Read the model definition and answer for the solid it produces. Units are mm, in the model's axes. Face numbers are marked on the shaded views. A direction names the side the tool comes from. Round coordinates to 2 decimals unless told otherwise and drop trailing zeros. Loops run counter-clockwise (first coordinate to the right, second up) from the corner with the lowest first, then second, coordinate; pieces in that order, holes last. Notation, with made-up numbers: (-14, -30.75) -> (8, -30.75) arc R25 ccw to (8, -17.75) -> close; hole circle Ø4 at (-25.5, 13.25). An arc over 180 degrees is marked (long way). Put each result on its own line as item: value.
from build123d import *

# Parameters (mm, degrees)
ESQUISSE1_W             = 77
ESQUISSE1_H             = 60
BOSS_EXTRU_1_DEPTH      = 3
BOSS_EXTRU_2_DEPTH      = 50
ESQUISSE3_W             = 55.4
ESQUISSE3_H             = 3
BOSS_EXTRU_3_DEPTH      = 74
ENL_V_MAT_EXTRU_2_REACH = 113.077
ESQUISSE5_R             = 5
BOSS_EXTRU_5_DEPTH      = 48
ENL_V_MAT_EXTRU_3_REACH = 113.077
ESQUISSE8_W             = 5
ESQUISSE8_H             = 10
ENL_V_MAT_EXTRU_4_DEPTH = 5
ESQUISSE10_R            = 5
ENL_V_MAT_EXTRU_5_DEPTH = 3
ESQUISSE11_W            = 74
ESQUISSE11_H            = 60
ENL_V_MAT_EXTRU_6_DEPTH = 5


with BuildPart() as part:
    # Esquisse1 → Boss.-Extru.1 (new body)
    with BuildSketch(Plane(origin=(0, 0, 0), x_dir=(1, 0, 0), z_dir=(0, 1, 0))):
        with Locations((38.5, 30)):
            Rectangle(ESQUISSE1_W, ESQUISSE1_H)
    extrude(amount=BOSS_EXTRU_1_DEPTH)

    # Esquisse2 → Boss.-Extru.2 (add)
    with BuildSketch(Plane(origin=(0, 3, 0), x_dir=(1, 0, 0), z_dir=(0, 1, 0))):
        Polygon((0, 60), (77, 60), (77, 0), (0, 0), (0, 2.3), (74, 2.3), (74, 57.7), (0, 57.7), align=None)
    extrude(amount=BOSS_EXTRU_2_DEPTH)

    # Esquisse3 → Boss.-Extru.3 (add)
    with BuildSketch(Plane.ZY.offset(-74)):
        with Locations((-30, 51.5)):
            Rectangle(ESQUISSE3_W, ESQUISSE3_H)
    extrude(amount=BOSS_EXTRU_3_DEPTH)

    # Esquisse5 → Enlèv. mat.-Extru.2 (cut, up to next)
    with BuildSketch(Plane(origin=(0, 0, -60), x_dir=(-1, 0, 0), z_dir=(0, 0, -1)), mode=Mode.PRIVATE) as enl_v_mat_extru_2_sk1:
        with Locations((-39, 29)):
            Circle(ESQUISSE5_R)
    enl_v_mat_extru_2_tool1 = extrude(enl_v_mat_extru_2_sk1.sketch, amount=-ENL_V_MAT_EXTRU_2_REACH, mode=Mode.PRIVATE) & part.part
    # Esquisse5 → Enlèv. mat.-Extru.2 (cut, up to next)
    with BuildSketch(Plane(origin=(0, 0, -60), x_dir=(-1, 0, 0), z_dir=(0, 0, -1)), mode=Mode.PRIVATE) as enl_v_mat_extru_2_sk2:
        with Locations((-10, 40.5)):
            Circle(ESQUISSE5_R)
    enl_v_mat_extru_2_tool2 = extrude(enl_v_mat_extru_2_sk2.sketch, amount=-ENL_V_MAT_EXTRU_2_REACH, mode=Mode.PRIVATE) & part.part
    add(enl_v_mat_extru_2_tool1.solids().sort_by_distance((39, 29, -60))[0], mode=Mode.SUBTRACT)
    add(enl_v_mat_extru_2_tool2.solids().sort_by_distance((10, 40.5, -60))[0], mode=Mode.SUBTRACT)

    # Esquisse7 → Boss.-Extru.5 (add)
    with BuildSketch(Plane.XZ):
        Polygon((0, 0), (-4.8, 0), (-4.8, -4.8), (-2.5, -4.8), (-2.5, -2.3), (0, -2.3), align=None)
        Polygon((0, -57.7), (0, -60), (-4.8, -60), (-4.8, -55.2), (-2.5, -55.2), (-2.5, -57.7), align=None)
    extrude(amount=-BOSS_EXTRU_5_DEPTH)

    # Esquisse8 → Enlèv. mat.-Extru.3 (cut, up to next)
    with BuildSketch(Plane(origin=(0, 53, 0), x_dir=(1, 0, 0), z_dir=(0, 1, 0)), mode=Mode.PRIVATE) as enl_v_mat_extru_3_sk1:
        with Locations((2.5, 30)):
            Rectangle(ESQUISSE8_W, ESQUISSE8_H)
    enl_v_mat_extru_3_tool1 = extrude(enl_v_mat_extru_3_sk1.sketch, amount=-ENL_V_MAT_EXTRU_3_REACH, mode=Mode.PRIVATE) & part.part
    add(enl_v_mat_extru_3_tool1.solids().sort_by_distance((2.5, 53, -30))[0], mode=Mode.SUBTRACT)

    # Esquisse9 → Enlèv. mat.-Extru.4 (cut)
    with BuildSketch(Plane.XZ):
        Polygon((0, -2.3), (-2.5, -2.3), (-2.5, -4.8), (-4.8, -4.8), (-4.8, 0), (0, 0), align=None)
        Polygon((0, -60), (0, -57.7), (-2.5, -57.7), (-2.5, -55.2), (-4.8, -55.2), (-4.8, -60), align=None)
    extrude(amount=-ENL_V_MAT_EXTRU_4_DEPTH, mode=Mode.SUBTRACT)

    # Esquisse10 → Enlèv. mat.-Extru.5 (cut)
    with BuildSketch(Plane.XY):
        with Locations((10, 12.5)):
            Circle(ESQUISSE10_R)
        with Locations((39, 24)):
            Circle(ESQUISSE10_R)
    extrude(amount=-ENL_V_MAT_EXTRU_5_DEPTH, mode=Mode.SUBTRACT)

    # Esquisse11 → Enlèv. mat.-Extru.6 (cut)
    with BuildSketch(Plane(origin=(0, 53, 0), x_dir=(1, 0, 0), z_dir=(0, 1, 0))):
        with Locations((37, 30)):
            Rectangle(ESQUISSE11_W, ESQUISSE11_H)
    extrude(amount=-ENL_V_MAT_EXTRU_6_DEPTH, mode=Mode.SUBTRACT)


solid = part.part
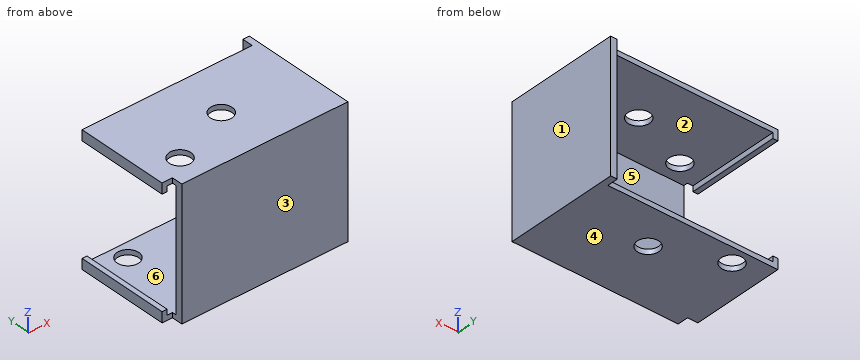
Item 1: The part is cut by section C-C (x = 57.5). Determine the outline of the cut face in (y, z).
Derived:
outline: (0, -60) -> (48, -60) -> (48, -57.7) -> (3, -57.7) -> (3, -2.3) -> (48, -2.3) -> (48, 0) -> (0, 0) -> close
Item 2: The part is cut by section D-D (y = 6). Determine the outline of the cut face in (x, z).
Derived:
outline: (-4.8, -60) -> (77, -60) -> (77, 0) -> (-4.8, 0) -> (-4.8, -4.8) -> (-2.5, -4.8) -> (-2.5, -2.3) -> (74, -2.3) -> (74, -57.7) -> (-2.5, -57.7) -> (-2.5, -55.2) -> (-4.8, -55.2) -> close
Item 3: Find the intervals of material crossed by line 1 along Z through (x, y) = (18, 35); line 2 along Y through (x, z) = (10, -58.5); line 3 along Y through (x, z) = (10, -0.55), in increasing order.
Derived:
line 1: z = -60 to -57.7, -2.3 to 0
line 2: y = 0 to 35.5, 45.5 to 48
line 3: y = 0 to 7.5, 17.5 to 48
Item 4: The part is cut by section B-B (x = 10). Determine the outline of the cut face in (y, z).
Derived:
outline: (0, -60) -> (35.5, -60) -> (35.5, -57.7) -> (3, -57.7) -> (3, -2.3) -> (7.5, -2.3) -> (7.5, 0) -> (0, 0) -> close; (17.5, -2.3) -> (48, -2.3) -> (48, 0) -> (17.5, 0) -> close; (45.5, -60) -> (48, -60) -> (48, -57.7) -> (45.5, -57.7) -> close
Item 5: For a pull along Z with two mould halves and no side action, classify the marked faces 3, 4, 5 and 6 as pulls with the +Z half, pulls with the -Z half, needs draft (parallel to the pull), parting line crosses it, or undercut.
Derived:
face 3: needs draft
face 4: pulls with the -Z half
face 5: undercut
face 6: undercut
Item 6: The part is cut by section A-A (y = 40.5). Determine the outline of the cut face in (x, z).
Derived:
outline: (-4.8, -60) -> (5, -60) -> (5, -57.7) -> (-2.5, -57.7) -> (-2.5, -55.2) -> (-4.8, -55.2) -> close; (-4.8, -4.8) -> (-2.5, -4.8) -> (-2.5, -2.3) -> (74, -2.3) -> (74, -57.7) -> (15, -57.7) -> (15, -60) -> (77, -60) -> (77, 0) -> (-4.8, 0) -> close
Item 7: Flat-ended cylindrical pins translate along their axes: pin 1 Ø1.5 at (x, z) = (9, -16) entering from +Y; pin 2 Ø4 at (y, z) = (2.5, -39.5) entering from -X; pin 3 Ø4 at (y, z) = (13, -7.5) entering from -X. Find the tip coordinate at first contact, or state that the pin passes through.
Derived:
pin 1: stops at y = 3
pin 2: stops at x = 0
pin 3: stops at x = 74
Item 8: Which of the six approach directions +Z, -Z, +X, -X, +Y, -Y give full straight-line access (tool end or side, diameter ignored) to the marked faces 1 and 2?
Derived:
face 1: +Z, -Z, +X, +Y, -Y
face 2: +Y
